For this review, use the dimensioned drawing (mm, ordinates from the lowest corner) and the shaded views. A direction names the side the tool comes from. Give positions to 0.01 mm unless a question says otherwise; leave off trailing zeros. Write each loop counter-clockwise with the first axis right and the second up, starting at its lowest first coordinate (ties: lowest second). Pieces come first, ordered by that corner, then holes. Notation, with made-up numbers: M -23.75,60.5 L -12.75,60.5 A17 cw -12.75,80.5 Z; hole C -2,71.5 d5. An arc over 180 degrees is marked long. Write each question's results on one line, items separated by ' | '. Start each with the question number.
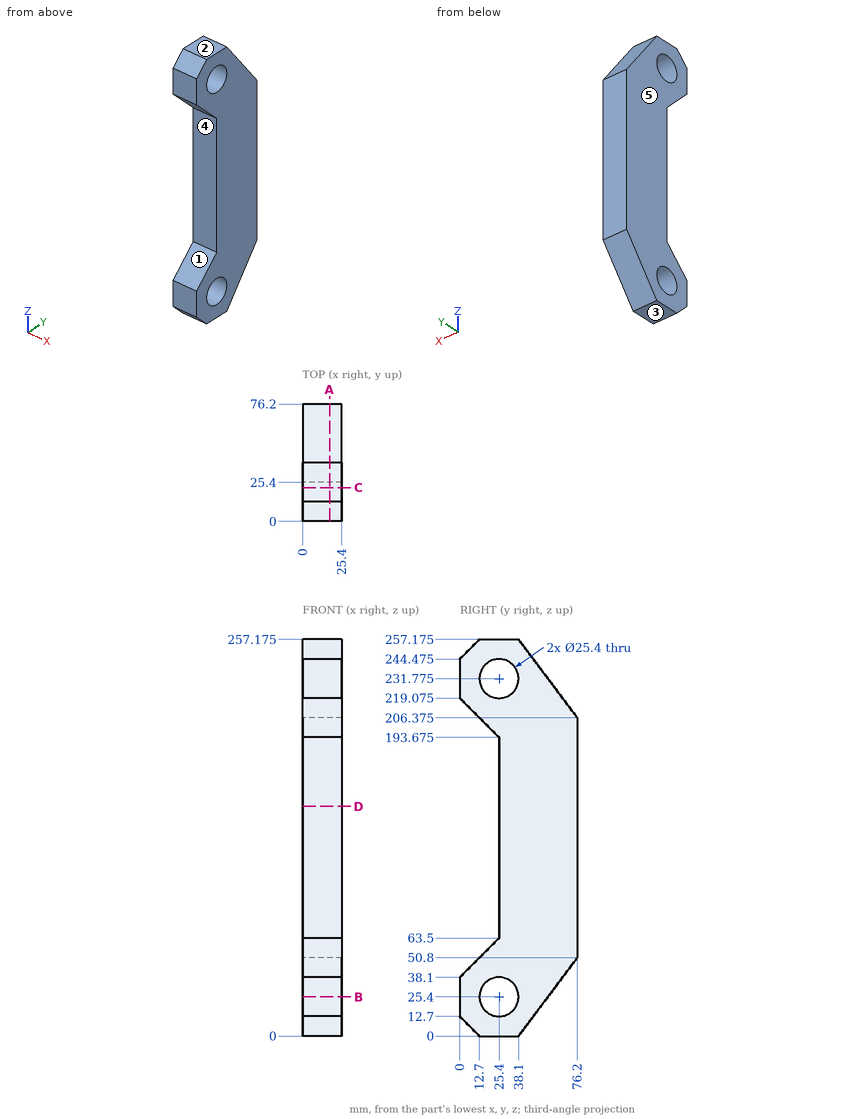
(1) Draft analysis for pull direction Z (two halves, no side actions). For the marked faces 1, 2 and 3, state which applies: pulls with the +Z half, pulls with the -Z half, needs draft (parallel to the pull), parting line crosses it, or undercut.
(2) Clearance check with flat-ended pins moving along their axes: P1, Ø12.5, axis at x = 14, z = 112.5, coming from the -Y side; P2, Ø3, axis at x = 14, z = 57, coming from the -Y side; P3, Ø23, axis at y = 25.4, z = 231.775, coming from the +X side. State where each tip first meets the part, or that it passes through.
(3) Machinability: for the marked faces 4 and 5, which of the approach directions +Z, -Z, +X, -X, +Y, -Y give a long, thin tool a straight path to every point of the face, cutting with its end or side? Answer none if there is none.
(4) Add section D-D (z = 149). State the section outline as (x, y) points.
(5) Add section B-B (z = 25.4). State the section outline as (x, y) points.
(6) Wall thickness on L1, parallel to Z at x = 3, y = 27 (3 decimals); L2, parallel to Z at x = 8.25, y = 35 (3 decimals); L3, parallel to Y at x = 16.75, z = 127.5: over which ranges is each line inside the solid? List them lowest first.
(7) Add section C-C (y = 22). State the section outline as (x, z) points (3 decimals).
(8) Add section A-A (x = 17.5). State the section outline as (y, z) points (3 decimals).
Calculated:
1) face 1: undercut | face 2: pulls with the +Z half | face 3: pulls with the -Z half
2) P1: stops at y = 25.4 | P2: stops at y = 17.4 | P3: passes through
3) face 4: +X, -X, -Y | face 5: +Z, -Z, -X, +Y, -Y
4) outline: M 0,25.4 L 25.4,25.4 L 25.4,76.2 L 0,76.2 Z
5) outline: M 0,0 L 25.4,0 L 25.4,12.7 L 0,12.7 Z; M 0,38.1 L 25.4,38.1 L 25.4,57.15 L 0,57.15 Z
6) L1: z = 0 to 12.801, 37.999 to 219.176, 244.374 to 257.175 | L2: z = 0 to 17.086, 33.714 to 223.461, 240.089 to 257.175 | L3: y = 25.4 to 76.2
7) outline: M 0,0 L 25.4,0 L 25.4,13.164 L 0,13.164 Z; M 0,37.636 L 25.4,37.636 L 25.4,60.1 L 0,60.1 Z; M 0,197.075 L 25.4,197.075 L 25.4,219.539 L 0,219.539 Z; M 0,244.011 L 25.4,244.011 L 25.4,257.175 L 0,257.175 Z
8) outline: M 0,12.7 L 12.7,0 L 38.1,0 L 76.2,50.8 L 76.2,206.375 L 38.1,257.175 L 12.7,257.175 L 0,244.475 L 0,219.075 L 25.4,193.675 L 25.4,63.5 L 0,38.1 Z; hole C 25.4,25.4 d25.4; hole C 25.4,231.775 d25.4
